Model file for the job. Use its own axes, mm. Round coordinates to 2 decimals unless told otherwise and drop trailing zeros. Order: outer loops, then holes, each group sorted by start corner. A loop starts at its lowest first (then second) coordinate and runs counter-clockwise, first axis right, second up. Notation, with made-up numbers: (38.5, -13) - (59.5, -13) arc R15 ccw to (59.5, -5) - close; hole circle Ø3 at (-35.5, -12.5). An arc over 180 degrees is marked (long way). Use one line per item in the form item = value.
from build123d import *

# Parameters (mm, degrees)
F0_R     = 12.5
F0_R_2   = 11
F1_DEPTH = 40
F2_R     = 11
F2_R_2   = 8.574422
F3_DEPTH = 29.8
F4_W     = 100
F4_H     = 11.153503
F5_DEPTH = 6


with BuildPart() as f1:
    # F0 (on Front) → F1 (new body, symmetric)
    with BuildSketch(Plane.XZ):
        Circle(F0_R)
        Circle(F0_R_2, mode=Mode.SUBTRACT)
    extrude(amount=F1_DEPTH, both=True)

    # F2 (on Front) → F3 (join, symmetric)
    with BuildSketch(Plane.XZ):
        Circle(F2_R)
        Circle(F2_R_2, mode=Mode.SUBTRACT)
    extrude(amount=F3_DEPTH, both=True)

    # F4 (on Top) → F5 (join, symmetric)
    with BuildSketch(Plane.XY):
        with Locations((-60.685454, -19.360414)):
            Rectangle(F4_W, F4_H)
        with Locations((60.685454, -19.360414)):
            Rectangle(F4_W, F4_H)
    extrude(amount=F5_DEPTH, both=True)


solid = f1.part
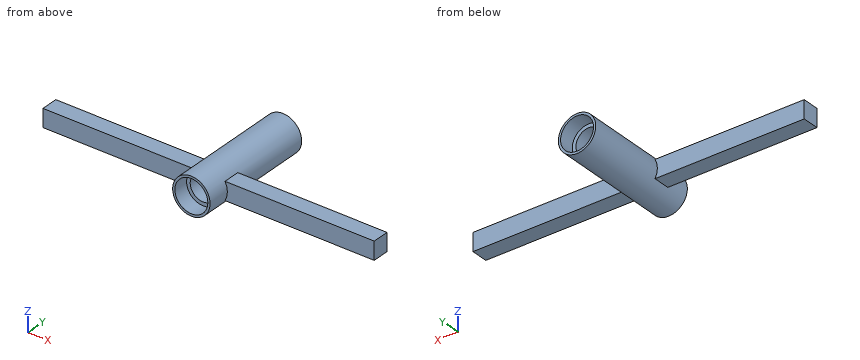
(1) Pin check, flat tips, straight feed: pin 1 (12.5 mm diameter, centred on x = -55, y = -21, fed in from +Z); pin 2 (12 mm diameter, centred on x = 7.5, y = 3, fed in from -Z); pin 3 (3.5 mm diameter, centred on x = 85.5, y = -20.5, fed in from -Z); pin 4 (6.5 mm diameter, centred on x = -2.5, z = -3, fed in from +Y). Stop position of each tip, or through.
Report:
pin_1 = 6
pin_2 = -12.41
pin_3 = -6
pin_4 = through
(2) Probe probe 1 along Z at (x, y) = (0, -36); probe 2 along X at (y, z) = (31, 0.5); probe 3 along Z at (x, y) = (0, -13). List the from-to ranges inside material, lowest first. Write a range as [from, to].
Report:
probe_1 = [-12.5, -11], [11, 12.5]
probe_2 = [-12.49, -10.99], [10.99, 12.49]
probe_3 = [-12.5, -8.57], [8.57, 12.5]
(3) Slice it at A-A on x = 0. Give the cut face in (y, z).
Report:
outline = (-40, -12.5) - (40, -12.5) - (40, -11) - (29.8, -11) - (29.8, -8.57) - (-29.8, -8.57) - (-29.8, -11) - (-40, -11) - close; (-40, 11) - (-29.8, 11) - (-29.8, 8.57) - (29.8, 8.57) - (29.8, 11) - (40, 11) - (40, 12.5) - (-40, 12.5) - close
(4) Slice it at B-B on z = 0. Give the cut face in (x, y).
Report:
outline = (-110.69, -24.94) - (-12.5, -24.94) - (-12.5, -40) - (-11, -40) - (-11, -29.8) - (-8.57, -29.8) - (-8.57, 29.8) - (-11, 29.8) - (-11, 40) - (-12.5, 40) - (-12.5, -13.78) - (-110.69, -13.78) - close; (8.57, -29.8) - (11, -29.8) - (11, -40) - (12.5, -40) - (12.5, -24.94) - (110.69, -24.94) - (110.69, -13.78) - (12.5, -13.78) - (12.5, 40) - (11, 40) - (11, 29.8) - (8.57, 29.8) - close
(5) Slice it at D-D on x = 34.5. Give the cut face in (y, z), then the cut area to 3 significant figures.
Report:
outline = (-24.94, -6) - (-13.78, -6) - (-13.78, 6) - (-24.94, 6) - close
area = 134 mm2
(6) Slice it at C-C on y = -34. Give the cut face in (x, z).
Report:
outline = circle Ø25 at (0, 0); hole circle Ø22 at (0, 0)
